Geometry check sheet. Reference: drawing and pictorial views, mm from the part's lowest x, y, z. Give positions to 0.01 mm unless a question says otherwise; leave off trailing zeros. Order: outer loops, then holes, each group sorted by start corner. A loop starts at its lowest first (then second) coordinate and runs counter-clockwise, first axis right, second up.
Item 1: Gauge pin test, flat ends, axial feed: P1, Ø1.5, axis at x = 45, y = 5, coming from the +Z side; P2, Ø3, axis at x = 43, y = 23, coming from the +Z side. Record the tip position at first contact, or that the pin passes through.
Item 2: Sectioned sample at C-C on z = 5. Record the boundary of the cut face in (x, y), and give its area (3 significant figures).
Item 3: Sectioned sample at B-B on y = 15. Record the boundary of the cut face in (x, z), and give its area (3 significant figures).
Item 4: Sectioned sample at D-D on y = 4.5. Record the boundary of the cut face in (x, z), and give its area (3 significant figures).
Item 5: Material ranges on line 1 along Y through (x, z) = (70, 20.5); line 2 along X through (y, z) = (14, 30); line 3 along X through (y, z) = (16, 42.5), recorded low to high.
Item 6: Release check for a two-part mould opening along Y. For the marked faces 1, 2, 3 and 4 record: released by +Y, released by -Y, zero draft, split by the parting line, or undercut.
Item 7: Sectioned sample at A-A on x = 70. Record the boundary of the cut face in (y, z), and give its area (3 significant figures).
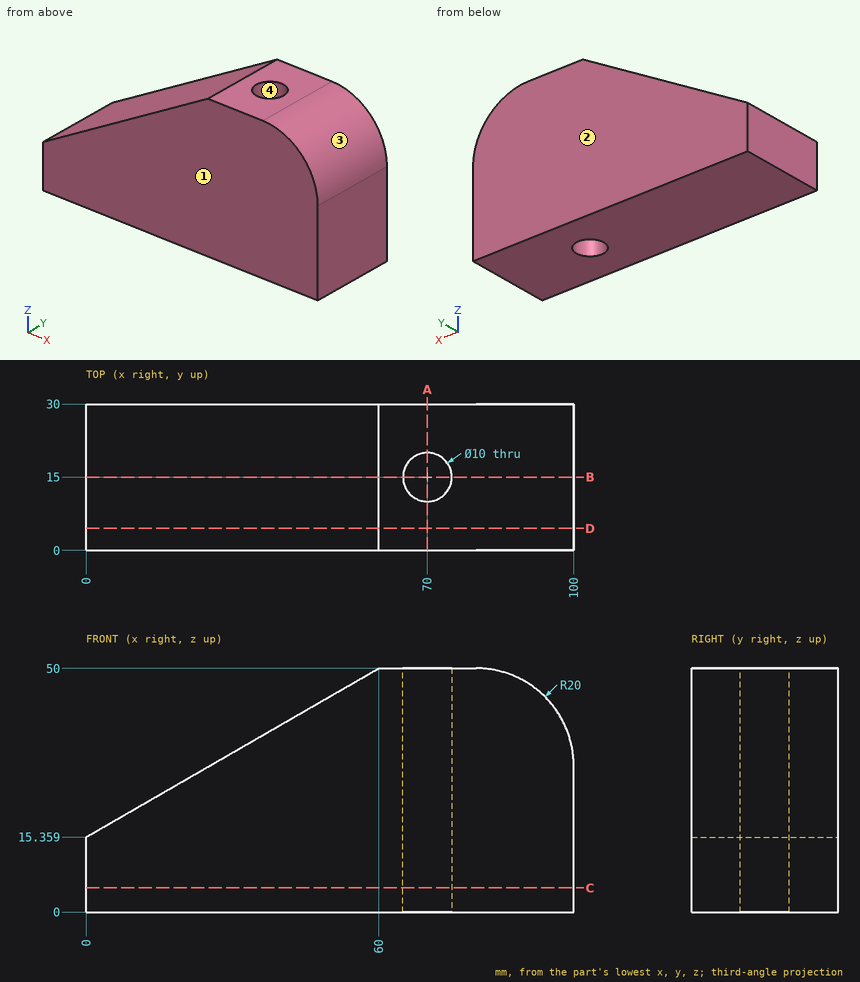
Report:
1. P1: stops at z = 41.77
1. P2: stops at z = 41.05
2. outline: (0, 0) - (100, 0) - (100, 30) - (0, 30) - close; hole circle Ø10 at (70, 15)
2. area: 2,920 mm2
3. outline: (0, 0) - (65, 0) - (65, 50) - (60, 50) - (0, 15.36) - close; (75, 0) - (100, 0) - (100, 30) arc R20 ccw to (80, 50) - (75, 50) - close
3. area: 3,370 mm2
4. outline: (0, 0) - (100, 0) - (100, 30) arc R20 ccw to (80, 50) - (60, 50) - (0, 15.36) - close
4. area: 3,870 mm2
5. line 1: y = 0 to 10, 20 to 30
5. line 2: x = 25.36 to 65.1, 74.9 to 100
5. line 3: x = 47.01 to 65.1, 74.9 to 95.61
6. face 1: released by -Y
6. face 2: released by +Y
6. face 3: zero draft
6. face 4: undercut
7. outline: (0, 0) - (10, 0) - (10, 50) - (0, 50) - close; (20, 0) - (30, 0) - (30, 50) - (20, 50) - close
7. area: 1,000 mm2
